Verification items for the finished model (mm, model axes). A direction names the side the tool comes from. Coordinates: 2 decimals unless noted, no trailing zeros. Write each loop counter-clockwise with the first axis right and the second up, starting at its lowest first coordinate (ties: lowest second). Pieces come first, ordered by that corner, then holes. Notation, with made-up numbers: (-19.75, 20) -> (-3.75, 20) arc R21 ccw to (-3.75, 55) -> close; hole circle Ø9 at (54.25, -14.75). An arc over 180 degrees is marked (long way). Use a Markdown table: item, result. Add a question column.
from build123d import *

# Parameters (mm, degrees)
BOSS_EXTRUDE1_DEPTH     = 15.875
CUT_EXTRUDE1_DEPTH      = 50.746098851
CUT_EXTRUDE1_DEPTH_BACK = 50.746098851
SKETCH3_R               = 3.2385
CUT_EXTRUDE2_DEPTH      = 81.103629898
CUT_EXTRUDE2_DEPTH_BACK = 81.103629898
SKETCH4_R               = 3.2385
SKETCH5_R               = 4.7625
CUT_EXTRUDE3_DEPTH      = 49.185254021


with BuildPart() as part:
    # Sketch1 → Boss-Extrude1 (new, symmetric)
    with BuildSketch(Plane.XY):
        with BuildLine():
            Line((50.8, 9.525), (50.8, -17.000540456))
            ThreePointArc((50.8, -17.000540456), (48.940128061, -21.490668516), (44.45, -23.350540456))
            ThreePointArc((44.45, -23.350540456), (43.211176455, -23.472553925), (42.019960204, -23.833905424))
            Line((42.019960204, -23.833905424), (27.353372626, -29.909004913))
            Line((27.353372626, -29.909004913), (24.92333283, -24.042369881))
            Line((24.92333283, -24.042369881), (41.483374135, -17.18297618))
            Line((41.483374135, -17.18297618), (21.098067328, 32.031507988))
            Line((21.098067328, 32.031507988), (26.964702359, 34.461547783))
            Line((26.964702359, 34.461547783), (33.039801848, 19.794960204))
            ThreePointArc((33.039801848, 19.794960204), (35.3785659, 16.945167962), (38.906436879, 15.875))
            Line((38.906436879, 15.875), (44.45, 15.875))
            ThreePointArc((44.45, 15.875), (48.940128061, 14.015128061), (50.8, 9.525))
        make_face()
    extrude(amount=BOSS_EXTRUDE1_DEPTH, both=True)

    # Sketch3 → Cut-Extrude1 (cut, two sides: drawn at the far end of the back side and taken through both)
    with BuildSketch(Plane(origin=(35.199810189, 14.580238773, 0), x_dir=(0, 0, -1), z_dir=(0.9238795325112886, 0.3826834323650853, 0)).offset(-CUT_EXTRUDE1_DEPTH_BACK)):
        with Locations(Location((-7.9375, 13.581873804, 0), (0, 0, 90))):
            Circle(SKETCH3_R)
        with Locations(Location((7.9375, 13.581873804, 0), (0, 0, 90))):
            Circle(SKETCH3_R)
        with BuildLine():
            Line((-15.875, 13.581873804), (-15.875, 21.519373804))
            Line((-15.875, 21.519373804), (-7.9375, 21.519373804))
            ThreePointArc((-7.9375, 21.519373804), (-13.550160076, 19.19453388), (-15.875, 13.581873804))
        make_face()
        with BuildLine():
            Line((7.9375, 21.519373804), (15.875, 21.519373804))
            Line((15.875, 21.519373804), (15.875, 13.581873804))
            ThreePointArc((15.875, 13.581873804), (13.550160076, 19.19453388), (7.9375, 21.519373804))
        make_face()
    extrude(amount=CUT_EXTRUDE1_DEPTH + CUT_EXTRUDE1_DEPTH_BACK, mode=Mode.SUBTRACT)

    # Sketch4 → Cut-Extrude2 (cut, two sides: drawn at the far end of the back side and taken through both)
    with BuildSketch(Plane(origin=(14.580238773, -35.199810189, 0), x_dir=(-0.9238795325112892, -0.3826834323650842, 0), z_dir=(0.3826834323650842, -0.9238795325112892, 0)).offset(-CUT_EXTRUDE2_DEPTH_BACK)):
        with Locations(Location((-21.763040456, -7.9375, 0), (0, 0, 180))):
            Circle(SKETCH4_R)
        with Locations(Location((-21.763040456, 7.9375, 0), (0, 0, 180))):
            Circle(SKETCH4_R)
        with BuildLine():
            Line((-13.825540456, -7.9375), (-13.825540456, -15.875))
            Line((-13.825540456, -15.875), (-21.763040456, -15.875))
            ThreePointArc((-21.763040456, -15.875), (-16.15038038, -13.550160076), (-13.825540456, -7.9375))
        make_face()
        with BuildLine():
            Line((-13.825540456, 7.9375), (-13.825540456, 15.875))
            Line((-13.825540456, 15.875), (-21.763040456, 15.875))
            ThreePointArc((-21.763040456, 15.875), (-16.15038038, 13.550160076), (-13.825540456, 7.9375))
        make_face()
    extrude(amount=CUT_EXTRUDE2_DEPTH + CUT_EXTRUDE2_DEPTH_BACK, mode=Mode.SUBTRACT)

    # Sketch5 → Cut-Extrude3 (cut, through all)
    with BuildSketch(Plane(origin=(50.8, 0, 0), x_dir=(0, 0, -1), z_dir=(1, 0, 0))):
        with Locations(Location((0, 0, 0), (0, 0, 90))):
            Circle(SKETCH5_R)
    extrude(amount=-CUT_EXTRUDE3_DEPTH, mode=Mode.SUBTRACT)


solid = part.part
1) Gauge pin test, flat ends, axial feed: pin 1 (1 mm diameter, centred on y = 4, z = -2, fed in from -X); pin 2 (8 mm diameter, centred on x = 46.5, z = -1, fed in from -Y); pin 3 (1.5 mm diameter, centred on y = 21, z = -11.5, fed in from -X); pin 4 (8 mm diameter, centred on y = -20, z = 7.5, fed in from +X). Record the tip position at first contact, or that the pin passes through.
2) Cross-section at C-C on z = -12. Record the boundary of the cut face in (x, y) (3 decimals), then the cut area to 3 significant figures.
3) Cross-section at B-B on y = -2.5. Record the boundary of the cut face in (x, z) (3 decimals).
4) Cross-section at D-D on x = 48. Record the boundary of the cut face in (y, z) (1 decimal), then the cut area to 3 significant figures.
5) Thickness scan on L1, parallel to Z at x = 46.75, y = 0 (1 decimal); L2, parallel to Y at x = 29.5, z = -7; L3, parallel to Y at x = 43, z = 0 (1 decimal). Record the ranges inside material, lowest first.
6) Release check for a two-part mould opening along Y. For faces 3 (the face through (28.327, -26.021, 13.612)), 4 (the face through (33.09, -20.66, 0.22)), 5 (the face through (24.904, 31.024, -13.612)), 6 (the face through (27.189, 25.507, -4.727)) record: released by +Y, released by -Y, zero draft, split by the parting line, or undercut.
7) Set-up check for faces 1 (the face through (24.86, 31.14, 13.49)), 2 (the face through (42, 15.875, 0)): record each of +Z, -Z, +X, -X, +Y, -Y from which the full face is reachable in a straight line by a thin tool's end or side.
Returned:
| question | item | result |
|---|---|---|
| 1 | pin 1 | stops at x = 32.5 |
| 1 | pin 2 | stops at y = -23.66 |
| 1 | pin 3 | stops at x = 25.36 |
| 1 | pin 4 | stops at x = 50.8 |
| 2 | outline | (21.526, 30.998) -> (41.483, -17.183) -> (25.957, -23.614) -> (28.387, -29.481) -> (42.02, -23.834) arc R6.35 cw to (44.45, -23.351) arc R6.35 ccw to (50.8, -17.001) -> (50.8, 9.525) arc R6.35 ccw to (44.45, 15.875) -> (38.906, 15.875) arc R6.35 cw to (33.04, 19.795) -> (27.393, 33.428) -> close |
| 2 | area | 789 mm² |
| 3 | outline | (35.401, -15.875) -> (50.8, -15.875) -> (50.8, -4.054) -> (35.401, -4.054) -> close; (35.401, 4.054) -> (50.8, 4.054) -> (50.8, 15.875) -> (35.401, 15.875) -> close |
| 4 | outline | (-22.3, -15.9) -> (14.8, -15.9) -> (14.8, 15.9) -> (-22.3, 15.9) -> close; hole circle Ø9.5 at (0, 0) |
| 4 | area | 1,110 mm² |
| 5 | L1 | z = -15.9 to -4.8, 4.8 to 15.9 |
| 5 | L2 | y = -29.02 to -22.45, 11.75 to 23.56 |
| 5 | L3 | y = -23.5 to -4.8, 4.8 to 15.9 |
| 6 | face 3 | released by -Y |
| 6 | face 4 | undercut |
| 6 | face 5 | released by +Y |
| 6 | face 6 | undercut |
| 7 | face 1 | +Z, -X, +Y |
| 7 | face 2 | +Z, -Z, +X, +Y |
